Read the model definition and answer for the solid it produces. Units are mm, in the model's axes. A direction names the side the tool comes from. Round coordinates to 2 decimals unless told otherwise and drop trailing zeros. Order: outer loops, then holes, each group sorted by start corner. A loop starts at its lowest first (then second) coordinate and runs counter-clockwise, first axis right, second up. Notation, with made-up numbers: (31, 13.5) - (47, 13.5) arc R28 ccw to (47, 51.5) - close; hole circle Ø2 at (-32, 29). An arc over 180 degrees is marked (long way). One line per question, with ' | ' between items. Start each with the question number.
1) The mould has two halves that part along X. Classify faces 1 (the cylindrical face through (47.655, 73.549, 11.591)), 2 (the cylindrical face through (-93.5, -27.4, 33)), 3 (the flat face through (-97, 1, 77)), 4 (the cylindrical face through (-86.473, 63.954, 40.56)): pulls with the +X half, pulls with the -X half, needs draft (parallel to the pull), parting line crosses it, or undercut.
2) Flat-ended cylindrical pins translate along their axes: pin 1 (7.5 mm diameter, centred on x = 93.5, z = 8.5, fed in from +Y); pin 2 (8 mm diameter, centred on x = 47, y = 53.5, fed in from +Z); pin 3 (5.5 mm diameter, centred on y = 4.5, z = 50, fed in from +X). Find the tip coordinate at first contact, or state that the pin passes through.
3) The part is cut by section C-C, the plane y = -47.5. Give the vertices of the cut face in (x, z).
4) Straight lines are drawn through the part: line 1 (Y direction, x = 66.5, z = -4.25); line 2 (X direction, y = -0.5, z = 16.5); line 3 (Y direction, x = 41, z = -3). For each, find the intervals that lie inside material, in ascending order. Write a range as from..to.
5) For faces 5 (the cylindrical face through (95.196, -75.289, 76.549)), 6 (the cylindrical face through (95.289, 75.196, 76.549)), 7 (the flat face through (1, 77, 31)), determine the directions among +Z, -Z, +X, -X, +Y, -Y from which every point of the face is accessible in a straight line to the end or side of a thin tool.
6) The part is cut by section A-A, the plane x = 2. Give the vertices of the cut face in (y, z).
7) The part is cut by section B-B, the plane z = 60.5. Give the vertices of the cut face in (x, y).
8) The part is cut by section D-D, the plane x = -77.5. Give the vertices of the cut face in (y, z).
from build123d import *

# Parameters (mm, degrees)
ESQUISSE1_R             = 5
BOSS_EXTRU_1_DEPTH      = 7
BOSS_EXTRU_2_START      = 80
ESQUISSE1_4_R           = 5
BOSS_EXTRU_2_DEPTH      = 80
CONG_1_R                = 2
ESQUISSE2_R             = 1.5
ENL_V_MAT_EXTRU_1_DEPTH = 80
ESQUISSE4_R             = 6.5
ENL_V_MAT_EXTRU_2_DEPTH = 10
ESQUISSE5_W             = 7
ESQUISSE5_H             = 14
ENL_V_MAT_EXTRU_3_DEPTH = 10
ENL_V_MAT_EXTRU_4_REACH = 213.492
ESQUISSE6_W             = 35
ESQUISSE6_H             = 3
ENL_V_MAT_EXTRU_5_REACH = 190.173
ESQUISSE7_W             = 3
ESQUISSE7_H             = 35
ENL_V_MAT_EXTRU_6_DEPTH = 10
BOSS_EXTRU_3_START      = 73
BOSS_EXTRU_3_DEPTH      = 3
CONG_2_R                = 2
ESQUISSE11_R            = 3
ENL_V_MAT_EXTRU_7_DEPTH = 10


with BuildPart() as part:
    # Esquisse1 → Boss.-Extru.1 (new body)
    with BuildSketch(Plane.XY):
        with BuildLine():
            Line((-91, -77), (91, -77))
            ThreePointArc((91, -77), (95.242640687, -75.242640687), (97, -71))
            Line((97, -71), (97, 71))
            ThreePointArc((97, 71), (95.242640687, 75.242640687), (91, 77))
            Line((91, 77), (-91, 77))
            ThreePointArc((-91, 77), (-95.242640687, 75.242640687), (-97, 71))
            Line((-97, 71), (-97, -71))
            ThreePointArc((-97, -71), (-95.242640687, -75.242640687), (-91, -77))
        make_face()
        with Locations((90, -70)):
            Circle(ESQUISSE1_R, mode=Mode.SUBTRACT)
        with Locations((90, 70)):
            Circle(ESQUISSE1_R, mode=Mode.SUBTRACT)
        with Locations((-90, 70)):
            Circle(ESQUISSE1_R, mode=Mode.SUBTRACT)
        with Locations((-90, -70)):
            Circle(ESQUISSE1_R, mode=Mode.SUBTRACT)
    extrude(amount=-BOSS_EXTRU_1_DEPTH)

    # Esquisse1<4> → Boss.-Extru.2 (add)
    with BuildSketch(Plane.XY.offset(BOSS_EXTRU_2_START)):
        with BuildLine():
            ThreePointArc((-97, -71), (-95.242640687, -75.242640687), (-91, -77))
            Line((-91, -77), (91, -77))
            ThreePointArc((91, -77), (95.242640687, -75.242640687), (97, -71))
            Line((97, -71), (97, 71))
            ThreePointArc((97, 71), (95.242640687, 75.242640687), (91, 77))
            Line((91, 77), (-91, 77))
            ThreePointArc((-91, 77), (-95.242640687, 75.242640687), (-97, 71))
            Line((-97, 71), (-97, -71))
        make_face()
        with Locations((-90, -70)):
            Circle(ESQUISSE1_4_R, mode=Mode.SUBTRACT)
        with BuildLine():
            ThreePointArc((-83, -70), (-85.050252532, -65.050252532), (-90, -63))
            Line((-90, -63), (-90, 63))
            ThreePointArc((-90, 63), (-85.050252532, 65.050252532), (-83, 70))
            Line((-83, 70), (83, 70))
            ThreePointArc((83, 70), (85.050252532, 65.050252532), (90, 63))
            Line((90, 63), (90, -63))
            ThreePointArc((90, -63), (85.050252532, -65.050252532), (83, -70))
            Line((83, -70), (-83, -70))
        make_face(mode=Mode.SUBTRACT)
        with Locations((90, -70)):
            Circle(ESQUISSE1_4_R, mode=Mode.SUBTRACT)
        with Locations((90, 70)):
            Circle(ESQUISSE1_4_R, mode=Mode.SUBTRACT)
        with Locations((-90, 70)):
            Circle(ESQUISSE1_4_R, mode=Mode.SUBTRACT)
    extrude(amount=-BOSS_EXTRU_2_DEPTH)

    # Congé1
    cong_1_edges = [part.edges().sort_by_distance(p)[0] for p in [
        (-83, -70, 40),
        (-90, -63, 40),
        (-90, 63, 40),
        (-83, 70, 40),
        (83, 70, 40),
        (90, 63, 40),
        (90, -63, 40),
        (83, -70, 40),
    ]]
    fillet(cong_1_edges, radius=CONG_1_R)

    # Esquisse2 → Enlèv. mat.-Extru.1 (cut)
    with BuildSketch(Plane.XY):
        with Locations((66.5, 28.5)):
            Circle(ESQUISSE2_R)
        with Locations((66.5, 63.5)):
            Circle(ESQUISSE2_R)
        with Locations((41.5, 63.5)):
            Circle(ESQUISSE2_R)
        with Locations((41.5, 28.5)):
            Circle(ESQUISSE2_R)
        with Locations((-10.5, 28.5)):
            Circle(ESQUISSE2_R)
        with Locations((14.5, 28.5)):
            Circle(ESQUISSE2_R)
        with Locations((-10.5, 63.5)):
            Circle(ESQUISSE2_R)
        with Locations((14.5, 63.5)):
            Circle(ESQUISSE2_R)
        with Locations((-62.5, 28.5)):
            Circle(ESQUISSE2_R)
        with Locations((-37.5, 28.5)):
            Circle(ESQUISSE2_R)
        with Locations((-62.5, 63.5)):
            Circle(ESQUISSE2_R)
        with Locations((-37.5, 63.5)):
            Circle(ESQUISSE2_R)
        with Locations((52.5, 1.5)):
            Circle(ESQUISSE2_R)
        with Locations((83.5, 1.5)):
            Circle(ESQUISSE2_R)
        with Locations((52.5, -19.5)):
            Circle(ESQUISSE2_R)
        with Locations((83.5, -19.5)):
            Circle(ESQUISSE2_R)
    extrude(amount=-ENL_V_MAT_EXTRU_1_DEPTH, mode=Mode.SUBTRACT)

    # Esquisse4 → Enlèv. mat.-Extru.2 (cut)
    with BuildSketch(Plane(origin=(0, 77, 0), x_dir=(1, 0, 0), z_dir=(0, 1, 0))):
        with Locations(Location((-50, -13, 0), (0, 0, 270))):
            Circle(ESQUISSE4_R)
        with Locations(Location((2, -13, 0), (0, 0, 270))):
            Circle(ESQUISSE4_R)
        with Locations(Location((54, -13, 0), (0, 0, 270))):
            Circle(ESQUISSE4_R)
    extrude(amount=-ENL_V_MAT_EXTRU_2_DEPTH, mode=Mode.SUBTRACT)

    # Esquisse5 → Enlèv. mat.-Extru.3 (cut)
    with BuildSketch(Plane(origin=(97, 0, 0), x_dir=(0, 0, -1), z_dir=(1, 0, 0))):
        with Locations((-9.5, -9)):
            Rectangle(ESQUISSE5_W, ESQUISSE5_H)
    extrude(amount=-ENL_V_MAT_EXTRU_3_DEPTH, mode=Mode.SUBTRACT)

    # Enlèv. mat.-Extru.4: up to this face of the body (flat: up to its plane)
    enl_v_mat_extru_4_end = Plane(part.part.faces().sort_by_distance((-90, 0, 40))[0])
    # Esquisse6 → Enlèv. mat.-Extru.4 (cut, up to the picked face)
    with BuildSketch(Plane(origin=(-83, 0, 0), x_dir=(0, 0, -1), z_dir=(1, 0, 0)), mode=Mode.PRIVATE) as enl_v_mat_extru_4_sk1:
        with Locations((-39.5, 66)):
            Rectangle(ESQUISSE6_W, ESQUISSE6_H)
    enl_v_mat_extru_4_tool1 = split(extrude(enl_v_mat_extru_4_sk1.sketch, amount=-ENL_V_MAT_EXTRU_4_REACH, mode=Mode.PRIVATE), bisect_by=enl_v_mat_extru_4_end, keep=Keep.BOTH, mode=Mode.PRIVATE)
    # Esquisse6 → Enlèv. mat.-Extru.4 (cut, up to the picked face)
    with BuildSketch(Plane(origin=(-83, 0, 0), x_dir=(0, 0, -1), z_dir=(1, 0, 0)), mode=Mode.PRIVATE) as enl_v_mat_extru_4_sk2:
        with Locations((-39.5, -66)):
            Rectangle(ESQUISSE6_W, ESQUISSE6_H)
    enl_v_mat_extru_4_tool2 = split(extrude(enl_v_mat_extru_4_sk2.sketch, amount=-ENL_V_MAT_EXTRU_4_REACH, mode=Mode.PRIVATE), bisect_by=enl_v_mat_extru_4_end, keep=Keep.BOTH, mode=Mode.PRIVATE)
    add(enl_v_mat_extru_4_tool1.solids().sort_by(Axis((-83, 66, 39.5), (-1, 0, 0)))[0], mode=Mode.SUBTRACT)
    add(enl_v_mat_extru_4_tool2.solids().sort_by(Axis((-83, -66, 39.5), (-1, 0, 0)))[0], mode=Mode.SUBTRACT)

    # Enlèv. mat.-Extru.5: up to this face of the body (flat: up to its plane)
    enl_v_mat_extru_5_end = Plane(part.part.faces().sort_by_distance((0, -70, 40))[0])
    # Esquisse7 → Enlèv. mat.-Extru.5 (cut, up to the picked face)
    with BuildSketch(Plane(origin=(0, -63, 0), x_dir=(1, 0, 0), z_dir=(0, 1, 0)), mode=Mode.PRIVATE) as enl_v_mat_extru_5_sk1:
        with Locations((86, -39.5)):
            Rectangle(ESQUISSE7_W, ESQUISSE7_H)
    enl_v_mat_extru_5_tool1 = split(extrude(enl_v_mat_extru_5_sk1.sketch, amount=-ENL_V_MAT_EXTRU_5_REACH, mode=Mode.PRIVATE), bisect_by=enl_v_mat_extru_5_end, keep=Keep.BOTH, mode=Mode.PRIVATE)
    add(enl_v_mat_extru_5_tool1.solids().sort_by(Axis((86, -63, 39.5), (0, -1, 0)))[0], mode=Mode.SUBTRACT)

    # Esquisse8 → Enlèv. mat.-Extru.6 (cut)
    with BuildSketch(Plane(origin=(0, -70, 0), x_dir=(1, 0, 0), z_dir=(0, 1, 0))):
        with BuildLine():
            ThreePointArc((-65.5, -42), (-65.939339828, -40.939339828), (-67, -40.5))
            Line((-67, -40.5), (-67, -42))
            Line((-67, -42), (-65.5, -42))
        make_face()
        with BuildLine():
            Line((-67, -42), (-67, -40.5))
            ThreePointArc((-67, -40.5), (-68.060660172, -43.060660172), (-65.5, -42))
            Line((-65.5, -42), (-67, -42))
        make_face()
        with BuildLine():
            Line((-67, -9.5), (-67, -8))
            Line((-67, -8), (-65.5, -8))
            ThreePointArc((-65.5, -8), (-68.060660172, -6.939339828), (-67, -9.5))
        make_face()
        with BuildLine():
            Line((-65.5, -8), (-67, -8))
            Line((-67, -8), (-67, -9.5))
            ThreePointArc((-67, -9.5), (-65.939339828, -9.060660172), (-65.5, -8))
        make_face()
        with BuildLine():
            ThreePointArc((-19.5, -8), (-21, -6.5), (-22.5, -8))
            Line((-22.5, -8), (-21, -8))
            Line((-21, -8), (-21, -9.5))
            ThreePointArc((-21, -9.5), (-19.939339828, -9.060660172), (-19.5, -8))
        make_face()
        with BuildLine():
            Line((-21, -8), (-22.5, -8))
            ThreePointArc((-22.5, -8), (-22.060660172, -9.060660172), (-21, -9.5))
            Line((-21, -9.5), (-21, -8))
        make_face()
        with BuildLine():
            ThreePointArc((-19.5, -42), (-19.939339828, -40.939339828), (-21, -40.5))
            Line((-21, -40.5), (-21, -42))
            Line((-21, -42), (-22.5, -42))
            ThreePointArc((-22.5, -42), (-21, -43.5), (-19.5, -42))
        make_face()
        with BuildLine():
            Line((-21, -42), (-21, -40.5))
            ThreePointArc((-21, -40.5), (-22.060660172, -40.939339828), (-22.5, -42))
            Line((-22.5, -42), (-21, -42))
        make_face()
    extrude(amount=-ENL_V_MAT_EXTRU_6_DEPTH, mode=Mode.SUBTRACT)

    # Esquisse10 → Boss.-Extru.3 (add)
    with BuildSketch(Plane.XY.offset(BOSS_EXTRU_3_START)):
        with BuildLine():
            Line((-94, -80), (94, -80))
            ThreePointArc((94, -80), (98.242640687, -78.242640687), (100, -74))
            Line((100, -74), (100, 74))
            ThreePointArc((100, 74), (98.242640687, 78.242640687), (94, 80))
            Line((94, 80), (-94, 80))
            ThreePointArc((-94, 80), (-98.242640687, 78.242640687), (-100, 74))
            Line((-100, 74), (-100, -74))
            ThreePointArc((-100, -74), (-98.242640687, -78.242640687), (-94, -80))
        make_face()
        with BuildLine():
            Line((-91, -77), (91, -77))
            ThreePointArc((91, -77), (95.242640687, -75.242640687), (97, -71))
            Line((97, -71), (97, 71))
            ThreePointArc((97, 71), (95.242640687, 75.242640687), (91, 77))
            Line((91, 77), (-91, 77))
            ThreePointArc((-91, 77), (-95.242640687, 75.242640687), (-97, 71))
            Line((-97, 71), (-97, -71))
            ThreePointArc((-97, -71), (-95.242640687, -75.242640687), (-91, -77))
        make_face(mode=Mode.SUBTRACT)
    extrude(amount=-BOSS_EXTRU_3_DEPTH)

    # Congé2
    cong_2_edges = [part.edges().sort_by_distance(p)[0] for p in [
        (97, 0, 70),
        (95.242640687, 75.242640687, 70),
        (0, 77, 70),
        (-95.242640687, 75.242640687, 70),
        (-97, 0, 70),
        (-95.242640687, -75.242640687, 70),
        (0, -77, 70),
        (95.242640687, -75.242640687, 70),
    ]]
    fillet(cong_2_edges, radius=CONG_2_R)

    # Esquisse11 → Enlèv. mat.-Extru.7 (cut)
    with BuildSketch(Plane(origin=(-90, 0, 0), x_dir=(0, 0, -1), z_dir=(1, 0, 0))):
        with Locations((-50, -27.5)):
            Circle(ESQUISSE11_R)
        with Locations((-50, 4.5)):
            Circle(ESQUISSE11_R)
        with Locations((-30, 4.5)):
            Circle(ESQUISSE11_R)
        with Locations((-30, -27.5)):
            Circle(ESQUISSE11_R)
    extrude(amount=-ENL_V_MAT_EXTRU_7_DEPTH, mode=Mode.SUBTRACT)


solid = part.part
Values:
1) face 1: undercut | face 2: needs draft | face 3: pulls with the -X half | face 4: undercut
2) pin 1: stops at y = 77 | pin 2: stops at z = 0 | pin 3: stops at x = 97
3) outline: (-100, 70) - (-99, 70) arc R2 cw to (-97, 68) - (-97, -7) - (97, -7) - (97, 68) arc R2 cw to (99, 70) - (100, 70) - (100, 73) - (97, 73) - (97, 80) - (90, 80) - (90, 0) - (-90, 0) - (-90, 80) - (-97, 80) - (-97, 73) - (-100, 73) - close
4) line 1: y = -77..27, 30..62, 65..77 | line 2: x = -97..-90, 90..97 | line 3: y = -77..27.09, 29.91..62.09, 64.91..77
5) face 5: +Z, +X, -Y | face 6: +Z, +X, +Y | face 7: -Z, +X, -X, +Y
6) outline: (-80, 70) - (-79, 70) arc R2 cw to (-77, 68) - (-77, -7) - (77, -7) - (77, 6.5) - (70, 6.5) - (70, 0) - (-70, 0) - (-70, 80) - (-77, 80) - (-77, 73) - (-80, 73) - close; (70, 19.5) - (77, 19.5) - (77, 68) arc R2 cw to (79, 70) - (80, 70) - (80, 73) - (77, 73) - (77, 80) - (70, 80) - close
7) outline: (-97, -71) arc R6 ccw to (-91, -77) - (91, -77) arc R6 ccw to (97, -71) - (97, 71) arc R6 ccw to (91, 77) - (-91, 77) arc R6 ccw to (-97, 71) - close; hole circle Ø10 at (-90, -70); hole circle Ø10 at (-90, 70); hole (-90, -61.23) arc R2 ccw to (-88.44, -63.18) arc R7 cw to (-83.18, -68.44) arc R2 ccw to (-81.23, -70) - (81.23, -70) arc R2 ccw to (83.18, -68.44) arc R7 cw to (88.44, -63.18) arc R2 ccw to (90, -61.23) - (90, 61.23) arc R2 ccw to (88.44, 63.18) arc R7 cw to (83.18, 68.44) arc R2 ccw to (81.23, 70) - (-81.23, 70) arc R2 ccw to (-83.18, 68.44) arc R7 cw to (-88.44, 63.18) arc R2 ccw to (-90, 61.23) - close; hole circle Ø10 at (90, -70); hole circle Ø10 at (90, 70)
8) outline: (-80, 70) - (-79, 70) arc R2 cw to (-77, 68) - (-77, -7) - (77, -7) - (77, 68) arc R2 cw to (79, 70) - (80, 70) - (80, 73) - (77, 73) - (77, 80) - (70, 80) - (70, 0) - (-70, 0) - (-70, 80) - (-77, 80) - (-77, 73) - (-80, 73) - close
